from build123d import *

# Parameters (mm, degrees)
F1_DEPTH = 38.1
F3_D     = 19.05
F5_D     = 19.05


with BuildPart() as f1:
    # F0 (on Front) → F1 (new body, symmetric)
    with BuildSketch(Plane.XZ):
        Polygon((-53.739256, 50.8), (-53.739256, 0), (73.260744, 0), (73.260744, 25.4), (22.470463, 25.4), (22.470463, 50.8), align=None)
    extrude(amount=F1_DEPTH, both=True)

    # F3 (through all)
    with Locations(Plane.YZ.offset(22.470463)):
        with Locations((0, 38.1)):
            Hole(F3_D / 2)

    # F5 (through all)
    with Locations(Plane.XY.offset(50.8)):
        with Locations((-15.634397, 0)):
            Hole(F5_D / 2)


solid = f1.part
Verification items for the finished model (mm, model axes). A direction names the side the tool comes from. Coordinates: 2 decimals unless noted, no trailing zeros. Order: outer loops, then holes, each group sorted by start corner. A loop starts at its lowest first (then second) coordinate and runs counter-clockwise, first axis right, second up. Notation, with made-up numbers: M 79.5,-29.75 L 135.5,-29.75 A21 cw 135.5,-10.75 Z; hole C 27,85.5 d7. An arc over 180 degrees is marked long. Return JSON: item names as keys, results as strings.
1) Access from +Z, -Z, +X, -X, +Y, -Y to the whole of each face (thin tool, end or side, straight path). Record for faces 5 (the flat face through (48, -1, 25.4)), 6 (the flat face through (73.261, -1, 13)).
Answer list:
{"face 5": "+Z, +X, +Y, -Y", "face 6": "+Z, -Z, +X, +Y, -Y"}
2) Cross-section at A-A, the plane y = 0. Record the boundary of the cut face in (x, z) (3 decimals), and give its area (3 significant figures).
Answer list:
{"outline": "M -53.739,0 L -25.159,0 L -25.159,28.575 L -53.739,28.575 Z; M -53.739,47.625 L -25.159,47.625 L -25.159,50.8 L -53.739,50.8 Z; M -6.109,0 L 73.261,0 L 73.261,25.4 L 22.47,25.4 L 22.47,28.575 L -6.109,28.575 Z; M -6.109,47.625 L 22.47,47.625 L 22.47,50.8 L -6.109,50.8 Z", "area": "3,100 mm2"}
3) Release check for a two-part mould opening along Y. For faces 1 (the flat face through (-5, -38.1, 20)), 2 (the flat face through (-5, 38.1, 20)), 3 (the cylindrical face through (-39.187, 9.516, 38.519)), 4 (the flat face through (9, -1, 0)) record: +Y half, -Y half, draft (parallel to the pull), parting line (faces both ways), or undercut.
Answer list:
{"face 1": "-Y half", "face 2": "+Y half", "face 3": "undercut", "face 4": "draft"}
4) Cross-section at C-C, the plane y = -17.5. Record the boundary of the cut face in (x, z).
Answer list:
{"outline": "M -53.74,0 L 73.26,0 L 73.26,25.4 L 22.47,25.4 L 22.47,50.8 L -53.74,50.8 Z"}
5) Gauge pin test, flat ends, axial feed: pin 1 (3 mm diameter, centred on y = -0.5, z = 30, fed in from +X); pin 2 (12 mm diameter, centred on x = 41, y = 18.5, fed in from +Z). Record the tip position at first contact, or that the pin passes through.
Answer list:
{"pin 1": "x = 22.47", "pin 2": "z = 25.4"}
6) Cross-section at D-D, the plane z = 33. Record the boundary of the cut face in (x, y) (3 decimals), and give its area (3 significant figures).
Answer list:
{"outline": "M -53.739,-38.1 L 22.47,-38.1 L 22.47,-8.045 L -10.534,-8.045 A9.525 cw -20.734,-8.045 L -53.739,-8.045 Z; M -53.739,8.045 L -20.734,8.045 A9.525 cw -10.534,8.045 L 22.47,8.045 L 22.47,38.1 L -53.739,38.1 Z", "area": "4,560 mm2"}
7) Cross-section at B-B, the plane z = 6. Record the boundary of the cut face in (x, y) (3 decimals), and give its area (3 significant figures).
Answer list:
{"outline": "M -53.739,-38.1 L 73.261,-38.1 L 73.261,38.1 L -53.739,38.1 Z; hole C -15.634,0 d19.05", "area": "9,390 mm2"}
8) Thickness scan on L1, parallel to Z at x = 5, y = 0 (3 decimals); L2, parallel to Z at x = 65.5, y = 16; L3, parallel to Y at x = -17.5, z = 32. Record the ranges inside material, lowest first. Write a range as [from, to].
Answer list:
{"L1": "[0, 28.575], [47.625, 50.8]", "L2": "[0, 25.4]", "L3": "[-38.1, -9.34], [9.34, 38.1]"}
